from build123d import *

# Parameters (mm, degrees)
F0_R     = 2.9972
F1_DEPTH = 22.225
F2_R     = 3.96875
F3_DEPTH = 12.7
F5_SIZE  = 0.508


with BuildPart() as f1:
    # F0 (on Top) → F1 (new body)
    with BuildSketch(Plane.XY):
        Circle(F0_R)
    extrude(amount=F1_DEPTH)


with BuildPart() as f3:
    # F2 (on Right) → F3 (new body, symmetric)
    with BuildSketch(Plane.YZ):
        with Locations((2.9972, 6.35)):
            Circle(F2_R)
    extrude(amount=F3_DEPTH, both=True)


with BuildPart() as f1_1:
    add(f1.part)

    # F4: cut F3
    add(f3.part, mode=Mode.SUBTRACT)

    # F5
    f5_edges = [f1_1.edges().sort_by_distance(p)[0] for p in [
        (-2.9972, 0, 22.225),
        (-2.9972, 0, 0),
    ]]
    chamfer(f5_edges, length=F5_SIZE)


solid = f1_1.part
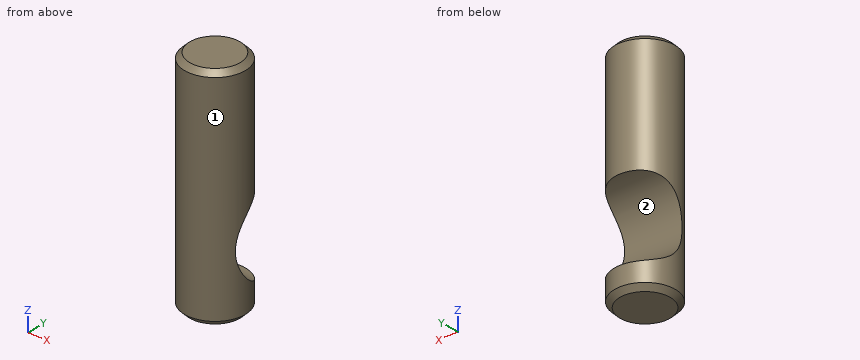
Could you check a few things on this model? Use its own coordinates, in mm. Face numbers are marked on the shaded views. Give positions to 0.01 mm unless a question says otherwise; leave off trailing zeros. Write each loop counter-clockwise with the first axis right and the second up, starting at its lowest first coordinate (ties: lowest second). Pieces come first, ordered by that corner, then holes. Notation, with made-up numbers: (-19, -38) -> (33, -38) arc R37 ccw to (33, -2) -> close; hole circle Ø1 at (27, -12). An arc over 180 degrees is marked (long way). Write each question's results on one line, items separated by ' | '. Start each with the question number.
Q1. We'd pull the mould along X, two halves only. Please class the marked faces 1 and 2: +X half, -X half, draft (parallel to the pull), parting line (faces both ways), or undercut.
Q2. I'm going to push a flat-ended pin straight in: pin 1 Ø1 at (x, z) = (-2, 5) entering from +Y. Where does the tip first touch, or does it pass through?
Q3. I need wall thicknesses on probe 1 along Z at (x, y) = (-0.75, -0.1) (3 decimals); probe 2 along Z at (x, y) = (-1.35, 2.2); probe 3 along X at (y, z) = (-2.25, 10.75). Which ranges of each line are inside material? Lowest first, please.
Q4. Suppose I cut it at C-C, the plane z = 20. List the corners of the cut face in (x, y) for me.
Q5. Suppose I cut it at A-A, the plane y = 0. List the corners of the cut face in (x, z) for me (1 decimal).
Q6. Suppose I cut it at D-D, the plane z = 6.35. List the corners of the cut face in (x, y) for me, and give its area (3 significant figures).
Outcome:
1) face 1: parting line | face 2: draft
2) pin 1: y = -0.51
3) probe 1: 0 to 3.868, 8.832 to 22.225 | probe 2: 0.09 to 2.46, 10.24 to 22.13 | probe 3: -1.98 to 1.98
4) outline: circle Ø5.99 at (0, 0)
5) outline: (-3, 0.5) -> (-2.5, 0) -> (2.5, 0) -> (3, 0.5) -> (3, 3.7) -> (-3, 3.7) -> close; (-3, 9) -> (3, 9) -> (3, 21.7) -> (2.5, 22.2) -> (-2.5, 22.2) -> (-3, 21.7) -> close
6) outline: (-2.84, -0.97) arc R3 ccw to (2.84, -0.97) -> close | area: 8.39 mm2
